Geometry check sheet. Reference: the model listing, model coordinates, mm. Round coordinates to 2 decimals unless told otherwise and drop trailing zeros. Loops run counter-clockwise (first coordinate to the right, second up) from the corner with the lowest first, then second, coordinate; pieces in that order, holes last. Notation, with made-up numbers: (72, 37.5) -> (77, 37.5) arc R10 ccw to (77, 47.5) -> close; hole circle Ø11 at (64.5, 70.5). An arc over 180 degrees is marked (long way). Use one line per item in the form item = value.
from build123d import *

# Parameters (mm, degrees)
F1_DEPTH = 25.4
F3_R     = 5.08


# Not quite as in the source:
# - a feature of the source that left no trace in its solid (it failed there, or was rolled back) is left out


with BuildPart() as f1:
    # F0 (on Front) → F1 (new body)
    with BuildSketch(Plane.XZ):
        Polygon((199.189722538, -57.2593323886), (-38.9998517931, 37.592638284), (0, 0), align=None)
    extrude(amount=F1_DEPTH)

    # F3
    f3_edges = [f1.edges().sort_by_distance(p)[0] for p in [
        (80.094935, -25.4, -9.833347),
        (-19.499926, -25.4, 18.796319),
        (99.594861, -25.4, -28.629666),
        (0, -12.7, 0),
        (199.189723, -12.7, -57.259332),
        (99.594861, 0, -28.629666),
        (80.094935, 0, -9.833347),
        (-19.499926, 0, 18.796319),
    ]]
    fillet(f3_edges, radius=F3_R)


solid = f1.part
1. Gauge pin test, flat ends, axial feed: pin 1 (10 mm diameter, centred on y = -9.5, z = 22, fed in from -X); pin 2 (5 mm diameter, centred on x = 55.5, y = -10, fed in from -Z); pin 3 (2 mm diameter, centred on x = 69.5, y = -17.5, fed in from -Z); pin 4 (12 mm diameter, centred on x = 69, z = -17.5, fed in from +Y). Record the tip position at first contact, or that the pin passes through.
Return value:
pin_1 = -28.01
pin_2 = -16.67
pin_3 = -20.27
pin_4 = 0
2. Material ranges on line 1 along Z through (x, y) = (77.5, -24); line 2 along Y through (x, z) = (-11.5, 22); line 3 along Y through (x, z) = (45, 0), recorded low to high.
Return value:
line_1 = -20.64 to -10.5
line_2 = -25.34 to -0.06
line_3 = -25.25 to -0.15
3. Section check A-A (y = -19). Record the boundary of the cut face in (x, z).
Return value:
outline = (-39, 37.59) -> (-0.91, 0.88) arc R5.08 ccw to (1.21, -0.35) -> (100.7, -28.95) arc R5.08 ccw to (103.98, -19.34) -> close
4. Mould release check, pull along Z, two halves, no side actions. Record for faces 1 (the cylindrical face through (-14.45, -1.53, 15.94)), 2 (the flat face through (25, -25.4, 1)), 3 (the flat face through (33.49, -12.593, 8.726)): released by +Z, released by -Z, zero draft, split by the parting line, or undercut.
Return value:
face_1 = released by -Z
face_2 = zero draft
face_3 = released by +Z
5. Section check B-B (y = -3). Record the boundary of the cut face in (x, z), then the cut area to 3 significant figures.
Return value:
outline = (-37.06, 36.34) -> (-0.6, 1.2) arc R4.63 ccw to (1.34, 0.08) -> (100.82, -28.52) arc R4.63 ccw to (103.81, -19.76) -> close
area = 2,000 mm2
